```python
from build123d import *
from build123d.topology import SkipClean

# Parameters (mm, degrees)
SKETCH1_R                   = 24
BOSS_EXTRUDE1_DEPTH         = 18
SKETCH2_R                   = 25.5
BOSS_EXTRUDE2_DEPTH         = 2
BOSS_EXTRUDE3_START         = -20
SKETCH2_2_R                 = 25.5
BOSS_EXTRUDE3_DEPTH         = 2
F_20_0MM_DOWEL_HOLE1_D      = 20
SKETCH13_R                  = 18
SKETCH13_R_2                = 10
BOSS_EXTRUDE4_DEPTH         = 8
SKETCH16_W                  = 1.65
SKETCH16_H                  = 25.5
TAP_DRILL_FOR_M4_TAP3_D     = 3.3
TAP_DRILL_FOR_M4_TAP3_DEPTH = 16.83
TAP_DRILL_FOR_M4_TAP3_TIP   = 0.991420021
TAP_DRILL_FOR_M4_TAP4_D     = 3.3
TAP_DRILL_FOR_M4_TAP4_DEPTH = 16.83
TAP_DRILL_FOR_M4_TAP4_TIP   = 0.991420021


with BuildPart() as part:
    # Sketch1 → Boss-Extrude1 (new body)
    with BuildSketch(Plane.XY):
        Circle(SKETCH1_R)
    extrude(amount=BOSS_EXTRUDE1_DEPTH)

    # Sketch2 → Boss-Extrude2 (add)
    with BuildSketch(Plane.XY.offset(18)):
        Circle(SKETCH2_R)
    extrude(amount=BOSS_EXTRUDE2_DEPTH)

    # Sketch2<2> → Boss-Extrude3 (add)
    with BuildSketch(Plane.XY.offset(18).offset(BOSS_EXTRUDE3_START)):
        Circle(SKETCH2_2_R)
    extrude(amount=BOSS_EXTRUDE3_DEPTH)

    # Ø20.0mm Dowel Hole1 (through all)
    with Locations(Plane.XY.offset(20)):
        with Locations((0, 0)):
            Hole(F_20_0MM_DOWEL_HOLE1_D / 2)

    # Sketch13 → Boss-Extrude4 (add)
    with SkipClean():  # the faces are left unmerged after this step: merging them gives an invalid solid
        with BuildSketch(Plane.XY.offset(20)):
            Circle(SKETCH13_R)
            Circle(SKETCH13_R_2, mode=Mode.SUBTRACT)
        extrude(amount=BOSS_EXTRUDE4_DEPTH)
    add(part.part.scale(1), mode=Mode.REPLACE)  # the faces are merged on a copy

    # Sketch16 → Tap Drill for M4 Tap1 (revolve, cut)
    with BuildSketch(Plane(origin=(0, 0, 24), x_dir=(0, 0, -1), z_dir=(1, 0, 0))):
        with Locations((0.825, 12.75)):
            Rectangle(SKETCH16_W, SKETCH16_H)
    revolve(axis=Axis((0, -6.35, 24), (0, 1, 0)), mode=Mode.SUBTRACT)

    # Tap Drill for M4 Tap3
    with Locations(Plane(origin=(-15.588457268, -9, 0), x_dir=(0, 0, -1), z_dir=(-0.8660254037844433, -0.49999999999999195, 0))):
        with Locations((-24, 0)):
            Hole(TAP_DRILL_FOR_M4_TAP3_D / 2, depth=TAP_DRILL_FOR_M4_TAP3_DEPTH)
            with Locations((0, 0, -(TAP_DRILL_FOR_M4_TAP3_DEPTH + TAP_DRILL_FOR_M4_TAP3_TIP / 2))):  # 118° drill point
                Cone(0, TAP_DRILL_FOR_M4_TAP3_D / 2, TAP_DRILL_FOR_M4_TAP3_TIP, mode=Mode.SUBTRACT)

    # Tap Drill for M4 Tap4
    with Locations(Plane(origin=(15.588457268, -9, 0), x_dir=(0, 0, -1), z_dir=(0.8660254037844364, -0.5000000000000041, 0))):
        with Locations((-24, 0)):
            Hole(TAP_DRILL_FOR_M4_TAP4_D / 2, depth=TAP_DRILL_FOR_M4_TAP4_DEPTH)
            with Locations((0, 0, -(TAP_DRILL_FOR_M4_TAP4_DEPTH + TAP_DRILL_FOR_M4_TAP4_TIP / 2))):  # 118° drill point
                Cone(0, TAP_DRILL_FOR_M4_TAP4_D / 2, TAP_DRILL_FOR_M4_TAP4_TIP, mode=Mode.SUBTRACT)


solid = part.part
```
CAD build for the part. Positions are in the model's coordinates, mm. A direction names the side the tool comes from. Coordinates: 2 decimals unless noted, no trailing zeros. Write each loop counter-clockwise with the first axis right and the second up, starting at its lowest first coordinate (ties: lowest second). Pieces come first, ordered by that corner, then holes.
(1) Cut at A-A, the plane y = 0. List the corners of the cut face in (x, z).
(2) Cut at C-C, the plane y = 17. List the corners of the cut face in (x, z).
(3) Two-plate mould, pull along Z, no slides. Class faces 1 (the face through (-5.5, -24.9, -1)), 2 (the face through (-23.977, 1.055, 8.874)), 3 (the face through (-17.4, -5.3, 20)): +Z half, -Z half, draft (parallel to the pull), parting line (faces both ways), or undercut.
(4) Cut at D-D, the plane x = 6. List the corners of the cut face in (y, z).
(5) Flat gauge pins, fed straight in: pin 1 (1.5 mm diameter, centred on y = 12, z = 24.5, fed in from -X); pin 2 (4 mm diameter, centred on x = 2.5, z = 6, fed in from -Y); pin 3 (12 mm diameter, centred on x = 0, y = 0, fed in from -Z); pin 4 (23 mm diameter, centred on x = 0, y = 0, fed in from +Z). Where does each tip first touch, or does it go through?
(6) Cut at B-B, the plane z = 24. List the corners of the cut face in (x, y).
(7) 3-axis set-ups, long thin cutter, end or side, ignore diameter. For faces 4 (the face through (15, -19, 18)), 5 (the face through (-2.343, 17.847, 23.944)), 6 (the face through (-0.07, 13.99, 25.65)), 7 (the face through (11, 0, -2)): which of +Z, -Z, +X, -X, +Y, -Y reach the whole face in a straight line?
(8) Drill centre lines: probe 1 along Z at (x, y) = (0, 14); probe 2 along Y at (x, z) = (0.5, 10); probe 3 along Y at (x, z) = (0.5, 21). Where is each one in solid material? Low to high.
Geometry says:
1. outline: (-25.5, -2) - (-10, -2) - (-10, 28) - (-18, 28) - (-18, 20) - (-25.5, 20) - (-25.5, 18) - (-24, 18) - (-24, 0) - (-25.5, 0) - close; (10, -2) - (25.5, -2) - (25.5, 0) - (24, 0) - (24, 18) - (25.5, 18) - (25.5, 20) - (18, 20) - (18, 28) - (10, 28) - close
2. outline: (-19.01, -2) - (19.01, -2) - (19.01, 0) - (16.94, 0) - (16.94, 18) - (19.01, 18) - (19.01, 20) - (5.92, 20) - (5.92, 28) - (-5.92, 28) - (-5.92, 20) - (-19.01, 20) - (-19.01, 18) - (-16.94, 18) - (-16.94, 0) - (-19.01, 0) - close; hole circle Ø3.3 at (0, 24)
3. face 1: draft
3. face 2: undercut
3. face 3: +Z half
4. outline: (-24.78, -2) - (-8, -2) - (-8, 28) - (-16.97, 28) - (-16.97, 20) - (-24.78, 20) - (-24.78, 18) - (-23.24, 18) - (-23.24, 0) - (-24.78, 0) - close; (8, -2) - (24.78, -2) - (24.78, 0) - (23.24, 0) - (23.24, 18) - (24.78, 18) - (24.78, 20) - (16.97, 20) - (16.97, 28) - (8, 28) - close
5. pin 1: stops at x = -14.05
5. pin 2: stops at y = -23.99
5. pin 3: passes through
5. pin 4: stops at z = 28
6. outline: (-16.35, -7.53) - (-9.37, -3.5) arc R10 cw to (-1.65, 9.86) - (-1.65, 17.92) arc R18 ccw to start; (-14.7, -10.39) arc R18 ccw to (14.7, -10.39) - (7.72, -6.36) arc R10 cw to (-7.72, -6.36) - close; (1.65, 9.86) arc R10 cw to (9.37, -3.5) - (16.35, -7.53) arc R18 ccw to (1.65, 17.92) - close
7. face 4: none
7. face 5: +Z
7. face 6: +Y
7. face 7: -Z, +X, -X, +Y, -Y
8. probe 1: z = -2 to 22.35, 25.65 to 28
8. probe 2: y = -23.99 to -9.99, 9.99 to 23.99
8. probe 3: y = -17.99 to -9.99, 9.99 to 17.99
